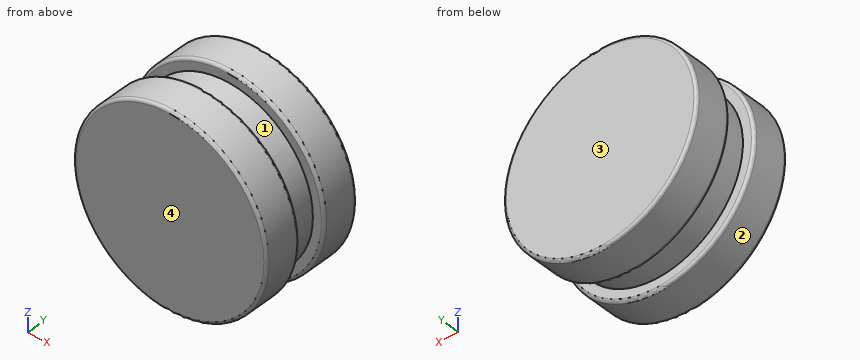
from build123d import *

# Parameters (mm, degrees)
SKETCH1_R           = 34.00044
BOSS_EXTRUDE1_DEPTH = 13
FILLET1_R           = 1
LPATTERN1_COUNT     = 2
LPATTERN1_PITCH     = 23.16
SKETCH2_R           = 30
BOSS_EXTRUDE2_DEPTH = 23.16


with BuildPart() as part:
    # Sketch1 → Boss-Extrude1 (new body)
    with BuildSketch(Plane(origin=(0, 0, 0), x_dir=(1, 0, 0), z_dir=(0, 1, 0))):
        Circle(SKETCH1_R)
    extrude(amount=BOSS_EXTRUDE1_DEPTH)

    # Fillet1
    fillet1_edges = [part.edges().sort_by_distance(p)[0] for p in [
        (-34.00044, 0, 0),
        (-34.00044, 13, 0),
    ]]
    fillet(fillet1_edges, radius=FILLET1_R)


with BuildPart() as lpattern1_1:
    # LPattern1: pattern copy
    add(part.part.moved(Location(Vector(0, 1, 0) * (1 * LPATTERN1_PITCH))))


with BuildPart() as part_1:
    add(part.part)

    add(lpattern1_1.part)  # Boss-Extrude2 merges LPattern1_1
    # Sketch2 → Boss-Extrude2 (add)
    with BuildSketch(Plane(origin=(0, 13, 0), x_dir=(1, 0, 0), z_dir=(0, 1, 0))):
        Circle(SKETCH2_R)
    extrude(amount=BOSS_EXTRUDE2_DEPTH)


solid = part_1.part
Here's how the part is built. I have some questions about the finished solid (model axes, mm). Face numbers are marked on the shaded views. Coordinates: 2 decimals unless noted, no trailing zeros. Order: outer loops, then holes, each group sorted by start corner. A loop starts at its lowest first (then second) coordinate and runs counter-clockwise, first axis right, second up. Notation, with made-up numbers: (70.5, 30.25) - (100.5, 30.25) arc R18 ccw to (100.5, 64.25) - close; hole circle Ø10 at (66.25, 20). An arc over 180 degrees is marked (long way). Use CSV: the item, a comma, the result in double quotes. Start each with the question number.
1. I'm going to push flat-ended pins straight in: pin 1 (4 mm diameter, centred on y = 17.5, z = 15.5, fed in from +X); pin 2 (2 mm diameter, centred on x = 24, y = 23.5, fed in from +Z); pin 3 (10 mm diameter, centred on y = 28.5, z = -19.5, fed in from -X). Where does each tip first touch, or does it pass through?
2. Suppose I cut it at C-C on y = 15. List the corners of the cut face in (x, z) for me.
3. Suppose I cut it at A-A on z = 0. List the corners of the cut face in (x, y) for me.
4. Please list where these lines run through material, in increasing order: line 1 (Y direction, x = 23, z = -20.5); line 2 (X direction, y = 2, z = -16); line 3 (Y direction, x = -17, z = -29). Write a range as from..to.
5. Suppose I cut it at D-D on y = 28. List the corners of the cut face in (x, z) for me.
6. Suppose I cut it at B-B on x = 0. List the corners of the cut face in (y, z) for me.
7. If we mould it in two halves opening along Y, with no side actions, what happens to the marked faces 1, 2, 3 and 4? For each: +Y half, -Y half, draft (parallel to the pull), parting line (faces both ways), or undercut.
Output:
1,pin 1,"stops at x = 26.79"
1,pin 2,"stops at z = 24.92"
1,pin 3,"stops at x = -30.75"
2,outline,"circle Ø60 at (0, 0)"
3,outline,"(-34, 1) arc R1 ccw to (-33, 0) - (33, 0) arc R1 ccw to (34, 1) - (34, 12) arc R1 ccw to (33, 13) - (30, 13) - (30, 23.16) - (33, 23.16) arc R1 ccw to (34, 24.16) - (34, 35.16) arc R1 ccw to (33, 36.16) - (-33, 36.16) arc R1 ccw to (-34, 35.16) - (-34, 24.16) arc R1 ccw to (-33, 23.16) - (-30, 23.16) - (-30, 13) - (-33, 13) arc R1 ccw to (-34, 12) - close"
4,line 1,"y = 0..13, 23.16..36.16"
4,line 2,"x = -30..30"
4,line 3,"y = 0.21..12.79, 23.37..35.95"
5,outline,"circle Ø68 at (0, 0)"
6,outline,"(0, -33) arc R1 ccw to (1, -34) - (12, -34) arc R1 ccw to (13, -33) - (13, -30) - (23.16, -30) - (23.16, -33) arc R1 ccw to (24.16, -34) - (35.16, -34) arc R1 ccw to (36.16, -33) - (36.16, 33) arc R1 ccw to (35.16, 34) - (24.16, 34) arc R1 ccw to (23.16, 33) - (23.16, 30) - (13, 30) - (13, 33) arc R1 ccw to (12, 34) - (1, 34) arc R1 ccw to (0, 33) - close"
7,face 1,"undercut"
7,face 2,"draft"
7,face 3,"+Y half"
7,face 4,"-Y half"
